Design review of the part built by this model. Coordinates are the model's own, in mm. Face numbers are marked on the shaded views. A direction names the side the tool comes from. Coordinates: 2 decimals unless noted, no trailing zeros. Loops run counter-clockwise (first coordinate to the right, second up) from the corner with the lowest first, then second, coordinate; pieces in that order, holes last. Notation, with made-up numbers: M -28,-14.5 L -15,-14.5 A6 cw -15,-3.5 Z; hole C 27,84.25 d5. An arc over 180 degrees is marked long. One line per item, written item: value.
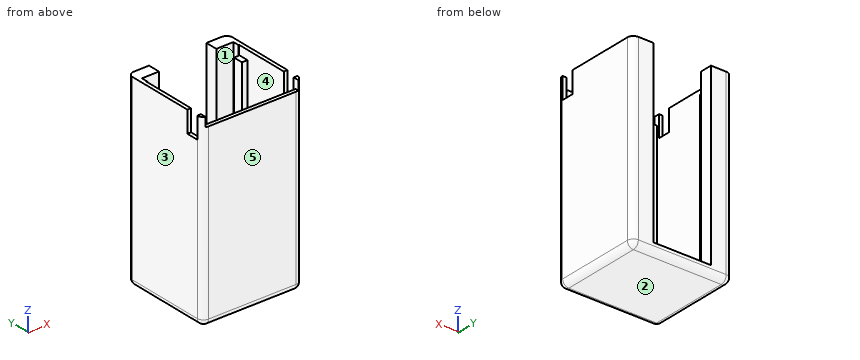
```python
from build123d import *

# Parameters (mm, degrees)
CROQUIS1_W              = 82
CROQUIS1_H              = 155
CROQUIS1_W_2            = 67
CROQUIS1_H_2            = 142.5
SALIENTE_EXTRUIR1_DEPTH = 5
CROQUIS1_3_W            = 82
CROQUIS1_3_H            = 155
CROQUIS1_3_W_2          = 67
CROQUIS1_3_H_2          = 142.5
SALIENTE_EXTRUIR2_DEPTH = 80
CROQUIS2_W              = 5
CROQUIS2_H              = 10
CROQUIS2_W_2            = 15
CORTAR_EXTRUIR1_DEPTH   = 120
CROQUIS4_W              = 75
CROQUIS4_H              = 5.5
CORTAR_EXTRUIR2_DEPTH   = 152.5
CROQUIS5_W              = 67
CROQUIS5_H              = 5
CORTAR_EXTRUIR4_DEPTH   = 140
CROQUIS6_W              = 147.5
CROQUIS6_H              = 15
SALIENTE_EXTRUIR3_DEPTH = 10
CORTAR_EXTRUIR5_DEPTH   = 147.5
CROQUIS7_3_W            = 17.5
CROQUIS7_3_H            = 5
CROQUIS7_3_W_2          = 64.5
CORTAR_EXTRUIR6_DEPTH   = 167.5
CROQUIS8_W              = 76
CROQUIS8_H              = 10
CORTAR_EXTRUIR7_DEPTH   = 60
CROQUIS9_W              = 82
CROQUIS9_H              = 2.5
CORTAR_EXTRUIR8_DEPTH   = 300
REDONDEO1_R             = 5


with BuildPart() as part:
    # Croquis1 → Saliente-Extruir1 (new body)
    with BuildSketch(Plane(origin=(0, 0, 0), x_dir=(1, 0, 0), z_dir=(0, 1, 0))):
        with Locations((0, 7.5)):
            Rectangle(CROQUIS1_W, CROQUIS1_H)
        with Locations((0, 6.25)):
            Rectangle(CROQUIS1_W_2, CROQUIS1_H_2, mode=Mode.SUBTRACT)
        with Locations((0, 6.25)):
            Rectangle(CROQUIS1_W_2, CROQUIS1_H_2)
    extrude(amount=SALIENTE_EXTRUIR1_DEPTH)

    # Croquis1_3 → Saliente-Extruir2 (add)
    with BuildSketch(Plane(origin=(0, 0, 0), x_dir=(1, 0, 0), z_dir=(0, 1, 0))):
        with Locations((0, 7.5)):
            Rectangle(CROQUIS1_3_W, CROQUIS1_3_H)
        with Locations((0, 6.25)):
            Rectangle(CROQUIS1_3_W_2, CROQUIS1_3_H_2, mode=Mode.SUBTRACT)
    extrude(amount=SALIENTE_EXTRUIR2_DEPTH)

    # Croquis2 → Cortar-Extruir1 (cut)
    with BuildSketch(Plane.ZY.offset(41)):
        with Locations((67.5, 10)):
            Rectangle(CROQUIS2_W, CROQUIS2_H)
        with Locations((57.5, 10)):
            Rectangle(CROQUIS2_W_2, CROQUIS2_H)
    extrude(amount=-CORTAR_EXTRUIR1_DEPTH, mode=Mode.SUBTRACT)

    # Croquis4 → Cortar-Extruir2 (cut)
    with BuildSketch(Plane.XY.offset(70)):
        with Locations((0, 62.25)):
            Rectangle(CROQUIS4_W, CROQUIS4_H)
    extrude(amount=-CORTAR_EXTRUIR2_DEPTH, mode=Mode.SUBTRACT)

    # Croquis5 → Cortar-Extruir4 (cut)
    with BuildSketch(Plane(origin=(0, 80, 0), x_dir=(1, 0, 0), z_dir=(0, 1, 0))):
        with Locations((0, -67.5)):
            Rectangle(CROQUIS5_W, CROQUIS5_H)
    extrude(amount=-CORTAR_EXTRUIR4_DEPTH, mode=Mode.SUBTRACT)

    # Croquis6 → Saliente-Extruir3 (add)
    with BuildSketch(Plane(origin=(-33.5, 0, 0), x_dir=(0, 0, -1), z_dir=(1, 0, 0))):
        with Locations((3.75, 72.5)):
            Rectangle(CROQUIS6_W, CROQUIS6_H)
    saliente_extruir3 = extrude(amount=SALIENTE_EXTRUIR3_DEPTH)

    # Simetr_a1: Saliente-Extruir3 across plane
    add(saliente_extruir3.mirror(Plane(origin=(0, 0, 0), x_dir=(0, 0, 1), z_dir=(1, 0, 0))))

    # Croquis7 → Cortar-Extruir5 (cut)
    with BuildSketch(Plane.XY.offset(70)):
        Polygon((-33.5, 51.5), (-38, 51.5), (-38, 3), (38, 3), (38, 51.5), align=None)
    extrude(amount=-CORTAR_EXTRUIR5_DEPTH, mode=Mode.SUBTRACT)

    # Croquis7_3 → Cortar-Extruir6 (cut)
    with BuildSketch(Plane.XY.offset(70)):
        with Locations((-32.25, 77.5)):
            Rectangle(CROQUIS7_3_W, CROQUIS7_3_H)
        with Locations((8.75, 77.5)):
            Rectangle(CROQUIS7_3_W_2, CROQUIS7_3_H)
    extrude(amount=-CORTAR_EXTRUIR6_DEPTH, mode=Mode.SUBTRACT)

    # Croquis8 → Cortar-Extruir7 (cut)
    with BuildSketch(Plane(origin=(0, 0, 0), x_dir=(-1, 0, 0), z_dir=(0, -1, 0))):
        with Locations((0, -65)):
            Rectangle(CROQUIS8_W, CROQUIS8_H)
    extrude(amount=-CORTAR_EXTRUIR7_DEPTH, mode=Mode.SUBTRACT)

    # Croquis9 → Cortar-Extruir8 (cut)
    with BuildSketch(Plane.XZ):
        with Locations((0, 68.75)):
            Rectangle(CROQUIS9_W, CROQUIS9_H)
    extrude(amount=-CORTAR_EXTRUIR8_DEPTH, mode=Mode.SUBTRACT)

    # Redondeo1
    redondeo1_edges = [part.edges().sort_by_distance(p)[0] for p in [
        (0, 75, -85),
        (41, 75, -8.75),
        (-41, 75, -8.75),
        (-41, 0, -8.75),
        (41, 0, -8.75),
        (0, 0, -85),
        (-41, 37.5, -85),
        (41, 37.5, -85),
    ]]
    fillet(redondeo1_edges, radius=REDONDEO1_R)


solid = part.part
```
(1) Insertion check: pin 1 (4 mm diameter, centred on x = 14.5, z = -57, fed in from +Y); pin 2 (3 mm diameter, centred on x = -21, y = 54, fed in from +Z); pin 3 (3.5 mm diameter, centred on x = -40, y = 8.5, fed in from +Z). Each pin has a flat end and moves straight along its axis. Give the tip position at first contact, or say it passes through.
Reply:
pin 1: stops at y = 3
pin 2: stops at z = -77.5
pin 3: stops at z = 50
(2) To check wall thickness, follow line 1 along Y through (x, z) = (35, -31); line 2 along X through (y, z) = (33.5, 9.5); line 3 along Y through (x, z) = (28.5, -54.5). State the ranges of each line that lie inside material, in increasing order. Write a range as [from, to].
Reply:
line 1: y = [0, 3], [51.5, 59.5], [65, 75]
line 2: x = [-41, -38], [38, 41]
line 3: y = [0, 3], [65, 75]
(3) We need section D-D on y = 8. State the section outline as (x, z) points, then the cut area to 3 significant figures.
Reply:
outline: M -41,-80 A5 ccw -36,-85 L 36,-85 A5 ccw 41,-80 L 41,50 L 38,50 L 38,-77.5 L -38,-77.5 L -38,50 L -41,50 Z
area: 1,370 mm2
(4) We need section C-C on z = 24.5. State the section outline as (x, y) points.
Reply:
outline: M -41,5 A5 ccw -36,0 L 36,0 A5 ccw 41,5 L 41,70 A5 ccw 36,75 L 23.5,75 L 23.5,65 L 37.5,65 L 37.5,59.5 L 33.5,59.5 L 33.5,51.5 L 38,51.5 L 38,3 L -38,3 L -38,51.5 L -33.5,51.5 L -33.5,59.5 L -37.5,59.5 L -37.5,65 L -23.5,65 L -23.5,75 L -36,75 A5 ccw -41,70 Z
(5) Tool access review of the marked faces 4 and 5: name each direction out of +Z, -Z, +X, -X, +Y, -Y from which nothing blocks a thin tool from reaching the whole face with its end or side.
Reply:
face 4: +Z
face 5: +Z, -Z, +X, -X, -Y
(6) We need section B-B on y = 63. State the section outline as (x, z) points, then the cut area to 3 significant figures.
Reply:
outline: M -41,-80 A5 ccw -36,-85 L 36,-85 A5 ccw 41,-80 L 41,67.5 L 37.5,67.5 L 37.5,-82.5 L -37.5,-82.5 L -37.5,67.5 L -41,67.5 Z
area: 1,240 mm2
(7) Mouldability with a two-part tool opening along X and no side actions: class the marked faces 1, 2 and 3 as released by +X, released by -X, zero draft, split by the parting line, or undercut.
Reply:
face 1: undercut
face 2: zero draft
face 3: released by -X
(8) We need section A-A on x = 9. State the section outline as (y, z) points, then the cut area to 3 significant figures.
Reply:
outline: M 0,-80 A5 ccw 5,-85 L 70,-85 A5 ccw 75,-80 L 75,-77.5 L 65,-77.5 L 65,-82.5 L 59.5,-82.5 L 59.5,-77.5 L 3,-77.5 L 3,60 L 0,60 Z
area: 937 mm2
